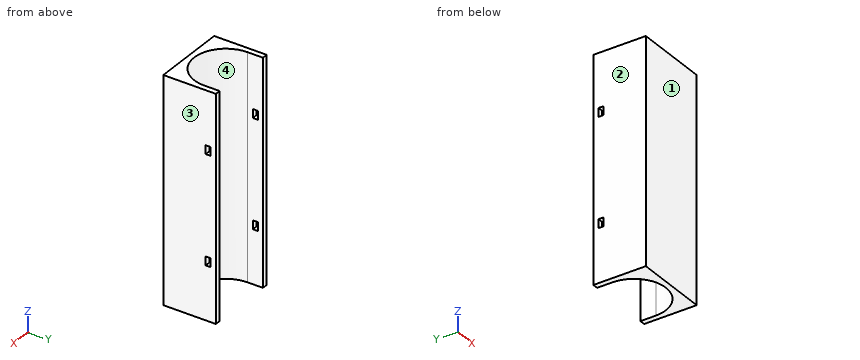
```python
from build123d import *

# Parameters (mm, degrees)
SKETCH1_W           = 76.2
SKETCH1_H           = 228.6
BOSS_EXTRUDE1_DEPTH = 38.1
SKETCH2_R           = 32.512
CUT_EXTRUDE2_DEPTH  = 244.959033446
SKETCH3_W           = 5.588
SKETCH3_H           = 15.705533419
BOSS_EXTRUDE2_DEPTH = 228.6
SKETCH4_W           = 8.89
SKETCH4_H           = 5.08
CUT_EXTRUDE3_DEPTH  = 247.899646469


with BuildPart() as part:
    # Sketch1 → Boss-Extrude1 (new body)
    with BuildSketch(Plane(origin=(0, 0, 0), x_dir=(1, 0, 0), z_dir=(0, 1, 0))):
        with Locations((38.1, 114.3)):
            Rectangle(SKETCH1_W, SKETCH1_H)
    extrude(amount=BOSS_EXTRUDE1_DEPTH)

    # Sketch2 → Cut-Extrude2 (cut, through all)
    with BuildSketch(Plane.XY):
        with Locations((38.1, 38.1)):
            Circle(SKETCH2_R)
    extrude(amount=-CUT_EXTRUDE2_DEPTH, mode=Mode.SUBTRACT)

    # Sketch3 → Boss-Extrude2 (add)
    with BuildSketch(Plane.XY):
        with Locations((2.794, 45.95276671)):
            Rectangle(SKETCH3_W, SKETCH3_H)
        with Locations((73.406, 45.95276671)):
            Rectangle(SKETCH3_W, SKETCH3_H)
    extrude(amount=-BOSS_EXTRUDE2_DEPTH)

    # Sketch4 → Cut-Extrude3 (cut, through all)
    with BuildSketch(Plane(origin=(76.2, 0, 0), x_dir=(0, 0, -1), z_dir=(1, 0, 0))):
        with Locations((59.055, 45.95276671)):
            Rectangle(SKETCH4_W, SKETCH4_H)
        with Locations((169.545, 45.95276671)):
            Rectangle(SKETCH4_W, SKETCH4_H)
    extrude(amount=-CUT_EXTRUDE3_DEPTH, mode=Mode.SUBTRACT)


solid = part.part
```
Could you check a few things on this model? Use its own coordinates, in mm. Face numbers are marked on the shaded views. Round coordinates to 2 decimals unless told otherwise and drop trailing zeros. Write each loop counter-clockwise with the first axis right and the second up, starting at its lowest first coordinate (ties: lowest second). Pieces come first, ordered by that corner, then holes. Notation, with made-up numbers: M 86.5,77 L 115.5,77 A25 cw 115.5,113 Z; hole C -7.5,-28 d3. An arc over 180 degrees is marked long. Write each question's results on one line, items separated by ' | '. Start each with the question number.
1. Imagine slicing it at C-C on z = -131.5. List the corners of the cut face in (x, y) for me, and give its area (3 significant figures).
2. Thinking about a two-plate mould opening in X: for the marked faces 1, 2, 3 and 4, which applies, +X half, -X half, draft (parallel to the pull), parting line (faces both ways), or undercut?
3. I need wall thicknesses on L1, parallel to X at y = 39, z = -140.5; L2, parallel to X at y = 13, z = -81.5; L3, parallel to Y at x = 37, z = -95. Which ranges of each line are inside material? Lowest first, please. Write a range as from..to.
4. Imagine slicing it at D-D on y = 32. List the corners of the cut face in (x, z) for me, and give its area (3 significant figures).
5. I'm going to push flat-ended pins straight in: pin 1 Ø5 at (x, z) = (57, -69) entering from +Y; pin 2 Ø12 at (x, z) = (28.5, -64.5) entering from +Y. Where does each tip first touch, or does it pass through?
6. Imagine slicing it at B-B on y = 14. List the corners of the cut face in (x, z) for me.
7. Imagine slicing it at A-A on z = -57.5. List the corners of the cut face in (x, y) for me.
Result sheet:
1) outline: M 0,0 L 76.2,0 L 76.2,53.81 L 70.61,53.81 L 70.61,38.1 A32.51 cw 5.59,38.1 L 5.59,53.81 L 0,53.81 Z | area: 1,420 mm^2
2) face 1: draft | face 2: -X half | face 3: +X half | face 4: undercut
3) L1: x = 0..5.59, 70.61..76.2 | L2: x = 0..17.44, 58.76..76.2 | L3: y = 0..5.61
4) outline: M 0,-228.6 L 6.17,-228.6 L 6.17,0 L 0,0 Z; M 70.03,-228.6 L 76.2,-228.6 L 76.2,0 L 70.03,0 Z | area: 2,820 mm^2
5) pin 1: stops at y = 13.62 | pin 2: stops at y = 9.58
6) outline: M 0,-228.6 L 16.28,-228.6 L 16.28,0 L 0,0 Z; M 59.92,-228.6 L 76.2,-228.6 L 76.2,0 L 59.92,0 Z
7) outline: M 0,0 L 76.2,0 L 76.2,43.41 L 70.61,43.41 L 70.61,38.1 A32.51 cw 5.59,38.1 L 5.59,43.41 L 0,43.41 Z; M 0,48.49 L 5.59,48.49 L 5.59,53.81 L 0,53.81 Z; M 70.61,48.49 L 76.2,48.49 L 76.2,53.81 L 70.61,53.81 Z
